Geometry check sheet. Reference: the model listing, model coordinates, mm. Round coordinates to 2 decimals unless told otherwise and drop trailing zeros. Loops run counter-clockwise (first coordinate to the right, second up) from the corner with the lowest first, then second, coordinate; pieces in that order, holes last.
```python
from build123d import *

# Parameters (mm, degrees)
BOSS_EXTRUDE1_DEPTH = 3
SKETCH2_R           = 1.6
CUT_EXTRUDE1_DEPTH  = 101.19374018
FILLET1_R           = 30
FILLET2_R           = 3


with BuildPart() as part:
    # Sketch1 → Boss-Extrude1 (new, symmetric)
    with BuildSketch(Plane(origin=(0, 0, 0), x_dir=(1, 0, 0), z_dir=(0, 1, 0))):
        Polygon((22.098076211, 0), (-22.098076211, 0), (-48.078838325, 15), (-98.882685902, 15), (-98.882685902, 9), (-49.686533479, 9), (-23.705771366, -6), (22.098076211, -6), align=None)
    extrude(amount=BOSS_EXTRUDE1_DEPTH, both=True)

    # Sketch2 → Cut-Extrude1 (cut, through all)
    with BuildSketch(Plane(origin=(0, 3, 0), x_dir=(1, 0, 0), z_dir=(0, 1, 0))):
        with Locations(Location((17.098076211, -3, 0), (0, 0, 270))):
            Circle(SKETCH2_R)
        with Locations(Location((-12.901923789, -3, 0), (0, 0, 270))):
            Circle(SKETCH2_R)
        with Locations(Location((-68.882685902, 12, 0), (0, 0, 270))):
            Circle(SKETCH2_R)
        with Locations(Location((-88.882685902, 12, 0), (0, 0, 270))):
            Circle(SKETCH2_R)
    extrude(amount=-CUT_EXTRUDE1_DEPTH, mode=Mode.SUBTRACT)

    # Fillet1
    fillet1_edges = [part.edges().sort_by_distance(p)[0] for p in [
        (-22.098076211, 0, 0),
        (-23.705771366, 0, 6),
        (-49.686533479, 0, -9),
        (-48.078838325, 0, -15),
    ]]
    fillet(fillet1_edges, radius=FILLET1_R)

    # Fillet2
    fillet2_edges = [part.edges().sort_by_distance(p)[0] for p in [
        (-98.882685902, 0, -9),
        (-98.882685902, 0, -15),
        (22.098076211, 0, 6),
        (22.098076211, 0, 0),
    ]]
    fillet(fillet2_edges, radius=FILLET2_R - 0.0001)  # a hair under: the kernel refuses the full size


solid = part.part
```
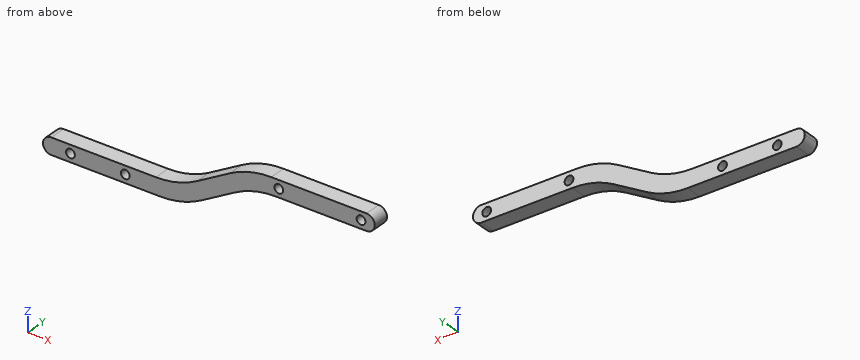
1) Sectioned sample at B-B, the plane x = -61. Record the cut outline in (y, z), then the cut area to 3 significant figures.
Report:
outline: (-3, -15) - (3, -15) - (3, -9) - (-3, -9) - close
area: 36.0 mm2
2) Sectioned sample at A-A, the plane y = 1. State how many separate pieces and enclosed holes the cut face has, then the cut area to 3 significant figures.
Report:
separate pieces: 1
enclosed holes: 4
area: 710 mm2
3) Sectioned sample at C-C, the plane z = -7.5. Record the cut outline in (x, y), then the cut area to 3 significant figures.
Report:
outline: (-48.36, -3) - (-35.09, -3) - (-35.09, 3) - (-48.36, 3) - close
area: 79.6 mm2
4) Gauge pin test, flat ends, axial feed: pin 1 (1 mm diameter, centred on x = -52.5, y = 1, fed in from -Z); pin 2 (5 mm diameter, centred on x = -88.88, z = -12, fed in from +Y); pin 3 (3 mm diameter, centred on x = -77.5, y = 0, fed in from +Z); pin 4 (3 mm diameter, centred on x = 5, y = -1.5, fed in from -Z). Record the tip position at first contact, or that the pin passes through.
Report:
pin 1: stops at z = -14.84
pin 2: stops at y = 3
pin 3: stops at z = -9
pin 4: stops at z = 0
5) Scan lines: line 1 along X through (y, z) = (-0.6, 3); line 2 along X through (y, z) = (0.75, -10.75); line 3 along Z through (x, y) = (6, 0.3). Record each from-to range of solid material in increasing order.
Report:
line 1: x = -28.74 to -14.5, -11.3 to 15.5, 18.7 to 22.1
line 2: x = -98.61 to -89.88, -87.88 to -69.88, -67.88 to -40.72
line 3: z = 0 to 6
